```python
from build123d import *

# Parameters (mm, degrees)
SKETCH1_W           = 80
SKETCH1_H           = 52
BOSS_EXTRUDE1_DEPTH = 8
SKETCH2_R           = 0.8
CUT_EXTRUDE2_DEPTH  = 5
SKETCH3_W           = 60.4
SKETCH3_H           = 40.4
CUT_EXTRUDE3_DEPTH  = 3.2
CHAMFER1_SIZE       = 1


with BuildPart() as part:
    # Sketch1 → Boss-Extrude1 (new body)
    with BuildSketch(Plane(origin=(33.5, 0, 0), x_dir=(0, 0, -1), z_dir=(1, 0, 0))):
        Rectangle(SKETCH1_W, SKETCH1_H)
    extrude(amount=BOSS_EXTRUDE1_DEPTH)

    # Sketch2 → Cut-Extrude2 (cut)
    with BuildSketch(Plane(origin=(33.5, 0, 0), x_dir=(0, 0, -1), z_dir=(1, 0, 0))):
        with Locations((-4.5, -4.5)):
            Circle(SKETCH2_R)
        with Locations((4.5, -4.5)):
            Circle(SKETCH2_R)
        with Locations((-4.5, 4.5)):
            Circle(SKETCH2_R)
        with Locations((4.5, 4.5)):
            Circle(SKETCH2_R)
    extrude(amount=CUT_EXTRUDE2_DEPTH, mode=Mode.SUBTRACT)

    # Sketch3 → Cut-Extrude3 (cut)
    with BuildSketch(Plane(origin=(41.5, 0, 0), x_dir=(0, 0, -1), z_dir=(1, 0, 0))):
        Rectangle(SKETCH3_W, SKETCH3_H)
    extrude(amount=-CUT_EXTRUDE3_DEPTH, mode=Mode.SUBTRACT)

    # Chamfer1
    chamfer1_edges = [part.edges().sort_by_distance(p)[0] for p in [
        (41.5, 26, 0),
        (41.5, -26, 0),
    ]]
    chamfer(chamfer1_edges, length=CHAMFER1_SIZE)


solid = part.part
```
CAD build for the part. Positions are in the model's coordinates, mm. A direction names the side the tool comes from. Coordinates: 2 decimals unless noted, no trailing zeros. Write each loop counter-clockwise with the first axis right and the second up, starting at its lowest first coordinate (ties: lowest second). Pieces come first, ordered by that corner, then holes. Notation, with made-up numbers: (68, -17.75) -> (118, -17.75) arc R18 ccw to (118, 8.25) -> close; hole circle Ø8 at (89, -14.75). An arc over 180 degrees is marked (long way). Return JSON: item names as keys, results as strings. Group by question number.
Q1. Which spindle directions (+Z, -Z, +X, -X, +Y, -Y) get a long thin tool onto all of the face, cutting with end or side? Do faces 1 (the face through (40, 20.2, 0)), 2 (the face through (37, -26, 1)). Say none if no direction does.
Q2. Drill centre lines: line 1 (Z direction, x = 36.95, y = -4.5); line 2 (Y direction, x = 37.1, z = 4.5); line 3 (Z direction, x = 40.75, y = -12). Where is each one in solid material? Low to high.
Q3. Cut at B-B, the plane y = 4.5. Give the cut face in (x, z), then the cut area to 3 significant figures.
Q4. Cut at C-C, the plane z = 25. Give the cut face in (x, y), then the cut area to 3 significant figures.
Q5. Flat gauge pins, fed straight in: pin 1 (1 mm diameter, centred on y = -4.5, z = -4.5, fed in from -X); pin 2 (10 mm diameter, centred on y = -17, z = -21.5, fed in from +X); pin 3 (1 mm diameter, centred on y = -19, z = -9.5, fed in from +X). Where does each tip first touch, or does it go through?
Q6. Cut at A-A, the plane z = 4.5. Give the cut face in (x, y), then the cut area to 3 significant figures.
Returned:
{
 "1": {"face 1": "+X", "face 2": "+Z, -Z, +X, -X, -Y"},
 "2": {"line 1": "z = -40 to -5.3, -3.7 to 3.7, 5.3 to 40", "line 2": "y = -26 to -5.3, -3.7 to 3.7, 5.3 to 26", "line 3": "z = -40 to -30.2, 30.2 to 40"},
 "3": {"outline": "(33.5, -40) -> (41.5, -40) -> (41.5, -30.2) -> (38.3, -30.2) -> (38.3, -5.3) -> (33.5, -5.3) -> close; (33.5, -3.7) -> (38.3, -3.7) -> (38.3, 3.7) -> (33.5, 3.7) -> close; (33.5, 5.3) -> (38.3, 5.3) -> (38.3, 30.2) -> (41.5, 30.2) -> (41.5, 40) -> (33.5, 40) -> close", "area": "431 mm2"},
 "4": {"outline": "(33.5, -26) -> (40.5, -26) -> (41.5, -25) -> (41.5, -20.2) -> (38.3, -20.2) -> (38.3, 20.2) -> (41.5, 20.2) -> (41.5, 25) -> (40.5, 26) -> (33.5, 26) -> close", "area": "286 mm2"},
 "5": {"pin 1": "passes through", "pin 2": "stops at x = 41.5", "pin 3": "stops at x = 38.3"},
 "6": {"outline": "(33.5, -26) -> (40.5, -26) -> (41.5, -25) -> (41.5, -20.2) -> (38.3, -20.2) -> (38.3, -5.3) -> (33.5, -5.3) -> close; (33.5, -3.7) -> (38.3, -3.7) -> (38.3, 3.7) -> (33.5, 3.7) -> close; (33.5, 5.3) -> (38.3, 5.3) -> (38.3, 20.2) -> (41.5, 20.2) -> (41.5, 25) -> (40.5, 26) -> (33.5, 26) -> close", "area": "270 mm2"}
}
